For this review, take the finished solid that the model builds, in its own axes (mm). Face numbers are marked on the shaded views. A direction names the side the tool comes from. Coordinates: 2 decimals unless noted, no trailing zeros. Loops run counter-clockwise (first coordinate to the right, second up) from the corner with the lowest first, then second, coordinate; pieces in that order, holes last. Notation, with made-up numbers: M 46,-15 L 80,-15 A23 cw 80,1 Z; hole C 73.5,-19 d9. An arc over 180 degrees is marked long. Answer as a JSON object with one key per item and string values. Group by question number.
Item 1: Tool access review of the marked faces 1 and 2: name each direction out of +Z, -Z, +X, -X, +Y, -Y from which nothing blocks a thin tool from reaching the whole face with its end or side.
Item 2: Add section C-C (y = 11.25). State the section outline as (x, z) points, then the cut area to 3 significant figures.
Item 3: Add section B-B (z = -17.5). State the section outline as (x, y) points, then the cut area to 3 significant figures.
Item 4: Add section A-A (x = 0). State the section outline as (y, z) points, then the cut area to 3 significant figures.
Item 5: Insertion check: pin 1 (4.5 mm diameter, centred on x = 15.16, z = 8.75, fed in from +Y); pin 2 (3 mm diameter, centred on x = -3.5, y = 4.5, fed in from -Z); pin 3 (8 mm diameter, centred on x = 9.5, z = 10, fed in from +Y). Each pin has a flat end and moves straight along its axis. Give the tip position at first contact, or say it passes through.
Item 6: Add section D-D (z = 0). State the section outline as (x, y) points.
Item 7: Mouldability with a two-part tool opening along Z and no side actions: class the marked faces 3, 4 and 5 as +Z half, -Z half, draft (parallel to the pull), parting line (faces both ways), or undercut.
Item 8: Wall thickness on L1, parallel to X at y = 2.75, z = 8.75; L2, parallel to Y at x = -12.5, z = 2; L3, parallel to Z at x = 3, y = 4: over which ranges is each line inside the solid? List them lowest first. Write a range as from..to.
from build123d import *

# Parameters (mm, degrees)
SKETCH1_R           = 1.75
SKETCH1_R_2         = 4.5
BOSS_EXTRUDE1_DEPTH = 6.35
FILLET1_R           = 5
SKETCH2_R           = 7
SKETCH2_R_2         = 4.5
BOSS_EXTRUDE2_DEPTH = 7.5
CHAMFER1_SIZE       = 5
CHAMFER1_SIZE2      = 3.372542584


with BuildPart() as part:
    # Sketch1 → Boss-Extrude1 (new body)
    with BuildSketch(Plane(origin=(0, 0, 0), x_dir=(1, 0, 0), z_dir=(0, 1, 0))):
        Polygon((-23.094010768, -13.333333333), (23.094010768, -13.333333333), (0, 26.666666667), align=None)
        with Locations(Location((0, 17.5, 0), (0, 0, 270))):
            Circle(SKETCH1_R, mode=Mode.SUBTRACT)
        with Locations(Location((-15.155444566, -8.75, 0), (0, 0, 270))):
            Circle(SKETCH1_R, mode=Mode.SUBTRACT)
        with Locations(Location((15.155444566, -8.75, 0), (0, 0, 270))):
            Circle(SKETCH1_R, mode=Mode.SUBTRACT)
        with Locations(Location((0, 0, 0), (0, 0, 270))):
            Circle(SKETCH1_R_2, mode=Mode.SUBTRACT)
    extrude(amount=BOSS_EXTRUDE1_DEPTH)

    # Fillet1
    fillet1_edges = [part.edges().sort_by_distance(p)[0] for p in [
        (-23.094010768, 3.175, 13.333333333),
        (0, 3.175, -26.666666667),
        (23.094010768, 3.175, 13.333333333),
    ]]
    fillet(fillet1_edges, radius=FILLET1_R)

    # Sketch2 → Boss-Extrude2 (add)
    with BuildSketch(Plane(origin=(0, 6.35, 0), x_dir=(1, 0, 0), z_dir=(0, 1, 0))):
        with Locations(Location((0, 0, 0), (0, 0, 270))):
            Circle(SKETCH2_R)
        with Locations(Location((0, 0, 0), (0, 0, 270))):
            Circle(SKETCH2_R_2, mode=Mode.SUBTRACT)
    extrude(amount=BOSS_EXTRUDE2_DEPTH)

    # Chamfer1
    chamfer1_edges = [part.edges().sort_by_distance(p)[0] for p in [
        (0, 6.35, -7),
    ]]
    chamfer1_side = [part.faces().sort_by_distance(p)[0] for p in [
        (0, 6.35, 12.810295705),
    ]]
    chamfer(chamfer1_edges, length=CHAMFER1_SIZE, length2=CHAMFER1_SIZE2, reference=chamfer1_side[0])


solid = part.part
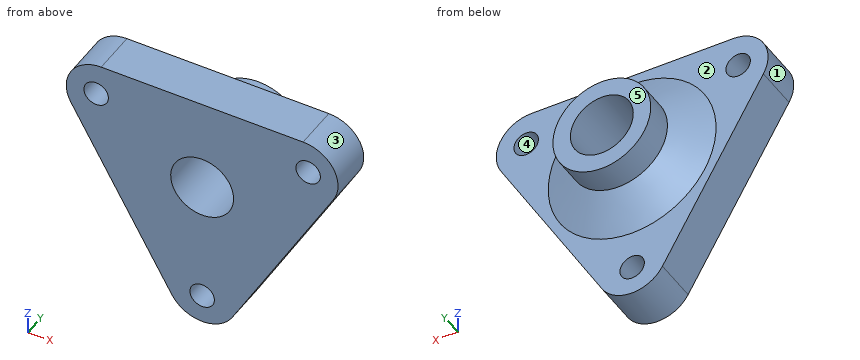
From the geometry:
{
 "1": {"face 1": "-X, +Y, -Y", "face 2": "+Y"},
 "2": {"outline": "C 0,0 d14; hole C 0,0 d9", "area": "90.3 mm²"},
 "3": {"outline": "M -5.29,0 L -1.75,0 L -1.75,6.35 L -5.29,6.35 Z; M 1.75,0 L 5.29,0 L 5.29,6.35 L 1.75,6.35 Z", "area": "45.0 mm²"},
 "4": {"outline": "M 0,-21.67 L 6.35,-21.67 L 6.35,-19.25 L 0,-19.25 Z; M 0,-15.75 L 6.35,-15.75 L 6.35,-12 L 9.72,-7 L 13.85,-7 L 13.85,-4.5 L 0,-4.5 Z; M 0,4.5 L 13.85,4.5 L 13.85,7 L 9.72,7 L 6.35,12 L 6.35,13.33 L 0,13.33 Z", "area": "197 mm²"},
 "5": {"pin 1": "stops at y = 6.35", "pin 2": "stops at z = -21.25", "pin 3": "stops at y = 7.84"},
 "6": {"outline": "M -15.4,0 L -4.5,0 L -4.5,13.85 L -7,13.85 L -7,9.72 L -12,6.35 L -15.4,6.35 Z; M 4.5,0 L 15.4,0 L 15.4,6.35 L 12,6.35 L 7,9.72 L 7,13.85 L 4.5,13.85 Z"},
 "7": {"face 3": "parting line", "face 4": "undercut", "face 5": "draft"},
 "8": {"L1": "x = -19.42..-16.91, -13.41..13.41, 16.91..19.42", "L2": "y = 0..6.35", "L3": "z = -20.67..-3.35, 3.35..13.33"}
}
